```python
from build123d import *

# Parameters (mm, degrees)
SKETCH1_W             = 117.475
SKETCH1_H             = 19.05
BOSS_EXTRUDE1_DEPTH   = 9.525
BOSS_EXTRUDE2_DEPTH   = 3.175
F_6_CLEARANCE_HOLE1_D = 4.3053
SKETCH5_W             = 12.065
SKETCH5_H             = 12.065
CUT_EXTRUDE1_DEPTH    = 10.525
SKETCH7_W             = 116.205
SKETCH7_H             = 14.605
CUT_EXTRUDE2_DEPTH    = 7.9502
SKETCH8_W             = 117.475
SKETCH8_H             = 28.575
CUT_EXTRUDE3_DEPTH    = 3.175
FILLET2_R             = 1.27
FILLET3_R             = 0.762
FILLET4_R             = 0.508


with BuildPart() as part:
    # Sketch1 → Boss-Extrude1 (new body)
    with BuildSketch(Plane.XY):
        with Locations((0, -57.6104797)):
            Rectangle(SKETCH1_W, SKETCH1_H)
    extrude(amount=BOSS_EXTRUDE1_DEPTH)

    # Sketch2 → Boss-Extrude2 (add)
    with BuildSketch(Plane.XY):
        with BuildLine():
            Line((35.56, -48.0854797), (58.7375, -48.0854797))
            Line((58.7375, -48.0854797), (44.939976119, -39.26086832))
            ThreePointArc((44.939976119, -39.26086832), (40.410479427, -39.106525106), (38.1, -43.0054797))
            Line((38.1, -43.0054797), (38.1, -45.5454797))
            ThreePointArc((38.1, -45.5454797), (37.356051224, -47.341530924), (35.56, -48.0854797))
        make_face()
        with BuildLine():
            Line((-38.1, -45.5454797), (-38.1, -43.0054797))
            ThreePointArc((-38.1, -43.0054797), (-40.410479427, -39.106525106), (-44.939976119, -39.26086832))
            Line((-44.939976119, -39.26086832), (-58.7375, -48.0854797))
            Line((-58.7375, -48.0854797), (-35.56, -48.0854797))
            ThreePointArc((-35.56, -48.0854797), (-37.356051224, -47.341530924), (-38.1, -45.5454797))
        make_face()
    extrude(amount=BOSS_EXTRUDE2_DEPTH)

    # #6 Clearance Hole1 (through all)
    with Locations(Plane.XY.offset(3.175)):
        with Locations((42.545, -43.0054797), (-42.545, -43.0054797)):
            Hole(F_6_CLEARANCE_HOLE1_D / 2)

    # Sketch5 → Cut-Extrude1 (cut, through all)
    with BuildSketch(Plane.XY.offset(9.525)):
        with Locations((50.8, -56.6198797)):
            Rectangle(SKETCH5_W, SKETCH5_H)
        with Locations((33.866666667, -56.6198797)):
            Rectangle(SKETCH5_W, SKETCH5_H)
        with Locations((16.933333333, -56.6198797)):
            Rectangle(SKETCH5_W, SKETCH5_H)
        with Locations((0, -56.6198797)):
            Rectangle(SKETCH5_W, SKETCH5_H)
        with Locations((-16.933333333, -56.6198797)):
            Rectangle(SKETCH5_W, SKETCH5_H)
        with Locations((-33.866666667, -56.6198797)):
            Rectangle(SKETCH5_W, SKETCH5_H)
        with Locations((-50.8, -56.6198797)):
            Rectangle(SKETCH5_W, SKETCH5_H)
    extrude(amount=-CUT_EXTRUDE1_DEPTH, mode=Mode.SUBTRACT)

    # Sketch7 → Cut-Extrude2 (cut)
    with BuildSketch(Plane(origin=(0, 0, 0), x_dir=(-1, 0, 0), z_dir=(0, 0, -1))):
        with Locations((0, -56.6198797)):
            Rectangle(SKETCH7_W, SKETCH7_H)
    extrude(amount=-CUT_EXTRUDE2_DEPTH, mode=Mode.SUBTRACT)

    # Sketch8 → Cut-Extrude3 (cut)
    with BuildSketch(Plane(origin=(0, 0, 0), x_dir=(-1, 0, 0), z_dir=(0, 0, -1))):
        with Locations((0, -52.8479797)):
            Rectangle(SKETCH8_W, SKETCH8_H)
    extrude(amount=-CUT_EXTRUDE3_DEPTH, mode=Mode.SUBTRACT)

    # Fillet2
    fillet2_edges = [part.edges().sort_by_distance(p)[0] for p in [
        (58.7375, -67.1354797, 6.35),
        (58.7375, -48.0854797, 6.35),
        (-58.7375, -48.0854797, 6.35),
        (-58.7375, -67.1354797, 6.35),
    ]]
    fillet(fillet2_edges, radius=FILLET2_R)

    # Fillet3
    fillet3_edges = [part.edges().sort_by_distance(p)[0] for p in [
        (-58.7375, -57.6104797, 9.525),
        (0, -48.0854797, 9.525),
        (0, -67.1354797, 9.525),
        (58.7375, -57.6104797, 9.525),
        (58.365525612, -66.763505312, 9.525),
        (58.365525612, -48.457454088, 9.525),
        (-58.365525612, -66.763505312, 9.525),
        (-58.365525612, -48.457454088, 9.525),
    ]]
    fillet(fillet3_edges, radius=FILLET3_R)

    # Fillet4
    fillet4_edges = [part.edges().sort_by_distance(p)[0] for p in [
        (0, -63.9223797, 7.9502),
        (-58.1025, -63.9223797, 5.5626),
        (-58.1025, -56.6198797, 7.9502),
        (-58.1025, -49.3173797, 5.5626),
        (0, -49.3173797, 7.9502),
        (58.1025, -49.3173797, 5.5626),
        (58.1025, -56.6198797, 7.9502),
        (58.1025, -63.9223797, 5.5626),
    ]]
    fillet(fillet4_edges, radius=FILLET4_R)


solid = part.part
```
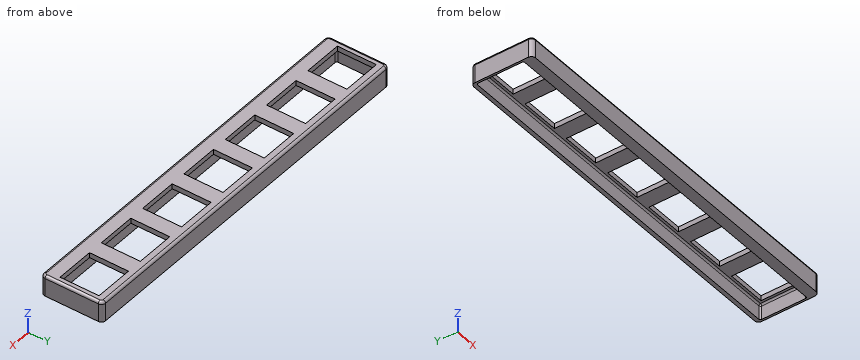
Input: part model. Units: mm. Frame: model coordinates. Coordinates: 2 decimals unless noted, no trailing zeros. Loops run counter-clockwise (first coordinate to the right, second up) from the corner with the lowest first, then second, coordinate; pieces in that order, holes last.
Q1. Section B-B, the plane z = 4.5. Return the cut outline in (x, y), and give its area (3 significant figures).
Results are:
outline: (-58.74, -65.87) arc R1.27 ccw to (-57.47, -67.14) - (57.47, -67.14) arc R1.27 ccw to (58.74, -65.87) - (58.74, -49.36) arc R1.27 ccw to (57.47, -48.09) - (-57.47, -48.09) arc R1.27 ccw to (-58.74, -49.36) - close; hole (-58.1, -63.41) arc R0.51 ccw to (-57.59, -63.92) - (57.59, -63.92) arc R0.51 ccw to (58.1, -63.41) - (58.1, -49.83) arc R0.51 ccw to (57.59, -49.32) - (-57.59, -49.32) arc R0.51 ccw to (-58.1, -49.83) - close
area: 540 mm2
Q2. Section C-C, the plane y = -56.75. Give the number of separate pieces and of enclosed holes in the cut face, and give its area (3 significant figures).
Results are:
separate pieces: 8
enclosed holes: 0
area: 57.9 mm2
Q3. Contact query for flat-ended pins moving along their axis: pin 1 (5 mm diameter, centred on x = -7, y = -56.5, fed in from -Z); pin 2 (2 mm diameter, centred on x = 16.5, y = -53, fed in from +Z). Output: stop coordinate, or through.
Results are:
pin 1: stops at z = 7.95
pin 2: passes through
Q4. Section A-A, the plane x = 50. Return the cut outline in (y, z) (3 decimals), and give its area (3 significant figures).
Results are:
outline: (-67.135, 3.175) - (-63.922, 3.175) - (-63.922, 7.442) arc R0.508 cw to (-63.414, 7.95) - (-62.652, 7.95) - (-62.652, 9.525) - (-66.373, 9.525) arc R0.762 ccw to (-67.135, 8.763) - close; (-50.587, 7.95) - (-49.825, 7.95) arc R0.508 cw to (-49.317, 7.442) - (-49.317, 3.175) - (-48.085, 3.175) - (-48.085, 8.763) arc R0.762 ccw to (-48.847, 9.525) - (-50.587, 9.525) - close
area: 32.1 mm2
Q5. Section D-D, the plane x = -26. Return the cut outline in (y, z) (3 decimals).
Results are:
outline: (-67.135, 3.175) - (-63.922, 3.175) - (-63.922, 7.442) arc R0.508 cw to (-63.414, 7.95) - (-49.825, 7.95) arc R0.508 cw to (-49.317, 7.442) - (-49.317, 3.175) - (-48.085, 3.175) - (-48.085, 8.763) arc R0.762 ccw to (-48.847, 9.525) - (-66.373, 9.525) arc R0.762 ccw to (-67.135, 8.763) - close
Q6. Line query: line 1 along Y through (x, z) = (12, 6); line 2 along X through (y, z) = (-59, 6.25); line 3 along Z through (x, y) = (24, -54) (3 decimals). Output: solid intervals per line, ascending.
Results are:
line 1: y = -67.14 to -63.92, -49.32 to -48.09
line 2: x = -58.74 to -58.1, 58.1 to 58.74
line 3: z = 7.95 to 9.525
